from build123d import *

# Parameters (mm, degrees)
F0_R     = 6.704343
F1_DEPTH = 76.2
F2_W     = 60.421344
F2_H     = 12.967138
F3_DEPTH = 7.62


with BuildPart() as f1:
    # F0 (on Right) → F1 (new body)
    with BuildSketch(Plane.YZ):
        Circle(F0_R)
    extrude(amount=F1_DEPTH)

    # F2 (on face) → F3 (join)
    with BuildSketch(Plane(origin=(0, 0, 0), x_dir=(0, -1, 0), z_dir=(-1, 0, 0))):
        Rectangle(F2_W, F2_H)
    extrude(amount=F3_DEPTH)


solid = f1.part
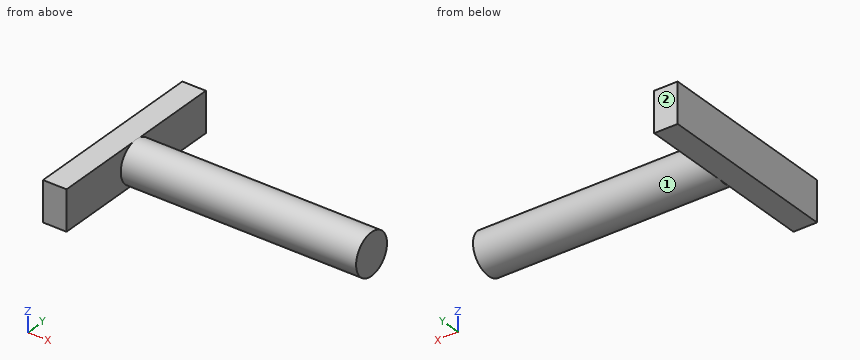
Part model, mm, in its own coordinate system. Face numbers are marked on the shaded views. A direction names the side the tool comes from. Give positions to 0.01 mm unless a question says otherwise; leave off trailing zeros. Loops run counter-clockwise (first coordinate to the right, second up) from the corner with the lowest first, then second, coordinate; pieces in that order, holes last.
(1) Band-saw the part on A-A (z = 0). Write the cut outline in (x, y), and give its area (3 significant figures).
Return value:
outline: (-7.62, -30.21) - (0, -30.21) - (0, -6.7) - (76.2, -6.7) - (76.2, 6.7) - (0, 6.7) - (0, 30.21) - (-7.62, 30.21) - close
area: 1,480 mm2
(2) Pin check, flat tips, straight feed: pin 1 (4 mm diameter, centred on y = 18.5, z = -2.5, fed in from +X); pin 2 (6 mm diameter, centred on x = 66.5, y = -11.5, fed in from +Z); pin 3 (6 mm diameter, centred on x = -2, y = -14.5, fed in from -Z); pin 4 (5 mm diameter, centred on x = 13.5, z = 3, fed in from -Y). Stop position of each tip, or through.
Return value:
pin 1: stops at x = 0
pin 2: passes through
pin 3: stops at z = -6.48
pin 4: stops at y = -6.69
(3) Drill centre lines: line 1 along Y through (x, z) = (18.5, 0.5); line 2 along X through (y, z) = (9, 2). Where is each one in solid material? Low to high.
Return value:
line 1: y = -6.69 to 6.69
line 2: x = -7.62 to 0
(4) Band-saw the part on D-D (z = 4). Write the cut outline in (x, y), and give its area (3 significant figures).
Return value:
outline: (-7.62, -30.21) - (0, -30.21) - (0, -5.38) - (76.2, -5.38) - (76.2, 5.38) - (0, 5.38) - (0, 30.21) - (-7.62, 30.21) - close
area: 1,280 mm2
(5) Band-saw the part on C-C (x = 23). Write the cut outline in (y, z).
Return value:
outline: circle Ø13.41 at (0, 0)
(6) 3-axis set-ups, long thin cutter, end or side, ignore diameter. For the marked faces 1 and 2: which of +Z, -Z, +X, -X, +Y, -Y reach the whole face in a straight line?
Return value:
face 1: +X
face 2: +Z, -Z, +X, -X, +Y
(7) Band-saw the part on B-B (y = -12). Write the cut outline in (x, z), and give its area (3 significant figures).
Return value:
outline: (-7.62, -6.48) - (0, -6.48) - (0, 6.48) - (-7.62, 6.48) - close
area: 98.8 mm2
